Print and shaded views of the part. All mm, measured from the part's lowest x, y and z. A direction names the side the tool comes from. Round coordinates to 2 decimals unless told otherwise and drop trailing zeros. Write each loop counter-clockwise with the first axis right and the second up, starting at its lowest first coordinate (ties: lowest second). Pieces come first, ordered by that corner, then holes. Notation, with made-up numbers: (53, 55.25) - (85, 55.25) arc R23 cw to (85, 86.25) - close; hole circle Ø5 at (74.5, 33.25). An arc over 180 degrees is marked (long way). Answer as a JSON object with one key per item and string values. Group by question number.
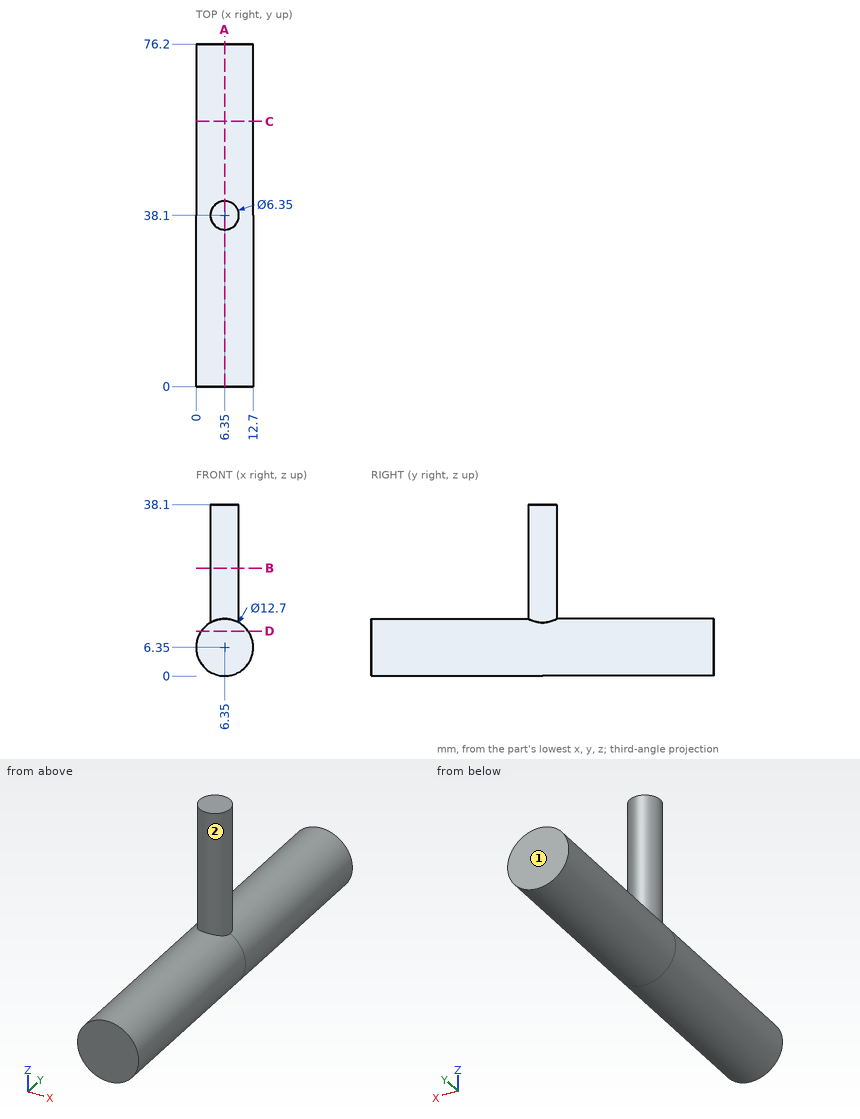
(1) Drill centre lines: line 1 (Z direction, x = 6, y = 46); line 2 (X direction, y = 26.5, z = 11). Where is each one in solid material? Low to high. Write a range as from..to.
(2) Slice it at B-B (z = 24). Write the cut outline in (x, y) (3 decimals).
(3) Slice it at C-C (y = 59). Write the cut outline in (x, z), then the cut area to 3 significant figures.
(4) Flat gauge pins, fed straight in: pin 1 (6 mm diameter, centred on x = 1.5, z = 32.5, fed in from -Y); pin 2 (1 mm diameter, centred on x = 9, y = 13.5, fed in from -Z); pin 3 (1.5 mm diameter, centred on x = 5.5, y = 31.5, fed in from +Z). Where does each tip first touch, or does it go through?
(5) Slice it at A-A (x = 6.35). Write the cut outline in (y, z) (3 decimals).
(6) 3-axis set-ups, long thin cutter, end or side, ignore diameter. For the marked faces 1 and 2: which of +Z, -Z, +X, -X, +Y, -Y reach the whole face in a straight line?
(7) Slice it at D-D (z = 10). Write the cut outline in (x, y), then the cut area to 3 significant figures.
Answer:
{
 "1": {"line 1": "0.01..12.69", "line 2": "2.03..10.67"},
 "2": {"outline": "circle Ø6.35 at (6.35, 38.1)"},
 "3": {"outline": "circle Ø12.7 at (6.35, 6.35)", "area": "127 mm²"},
 "4": {"pin 1": "y = 35.52", "pin 2": "z = 0.38", "pin 3": "z = 12.7"},
 "5": {"outline": "(0, 0) - (76.2, 0) - (76.2, 12.7) - (41.275, 12.7) - (41.275, 38.1) - (34.925, 38.1) - (34.925, 12.7) - (0, 12.7) - close"},
 "6": {"face 1": "+Z, -Z, +X, -X, +Y", "face 2": "+Z"},
 "7": {"outline": "(1.15, 0) - (11.55, 0) - (11.55, 76.2) - (1.15, 76.2) - close", "area": "792 mm²"}
}
